The listing builds one solid part. Answer for the finished solid, in the listing's coordinates (mm). Face numbers are marked on the shaded views. A direction names the side the tool comes from. Round coordinates to 2 decimals unless told otherwise and drop trailing zeros. Write each loop counter-clockwise with the first axis right and the second up, starting at its lowest first coordinate (ties: lowest second). Pieces come first, ordered by that corner, then holes. Notation, with made-up numbers: (-6.75, 37.25) - (-1.75, 37.25) arc R31 cw to (-1.75, 64.25) - close; hole circle Ø2 at (20.25, 26.25). An arc over 180 degrees is marked (long way). Use a Markdown table: item, result. Add a question column.
1) A tool of negligible diameter and unlimited length cuts with its end or side. For the marked faces 1 and 2, from which of +Z, -Z, +X, -X, +Y, -Y can it reach the whole face along a straight path? Write none if from no direction.
2) Each of these flat-tipped pins is pushed along its axis until it touches: P1, Ø1, axis at x = 38.5, y = 7, coming from the +Z side; P2, Ø1.5, axis at y = 34, z = -273, coming from the +X side. Where does it stop, or does it pass through?
3) Find the intervals of material crossed by probe 1 along X at (y, z) = (30, -216); probe 2 along Z at (x, y) = (-120, 26.5) (3 decimals), in increasing order. Write a range as from..to.
4) A cutting plane is placed at A-A (x = -148). Give the vertices of the cut face in (y, z) (3 decimals), then the cut area to 3 significant figures.
5) A cutting plane is placed at B-B (z = -319.5). Give the vertices of the cut face in (x, y) (1 decimal), then the cut area to 3 significant figures.
```python
from build123d import *

# Parameters (mm, degrees)
SKETCH1_W           = 473.075
SKETCH1_H           = 95.25
BOSS_EXTRUDE1_DEPTH = 3.175
SKETCH3_W           = 78.74
SKETCH3_H           = 51.308
CUT_EXTRUDE2_DEPTH  = 242.305221983
SKETCH4_R           = 8.255
CUT_EXTRUDE3_DEPTH  = 242.305221983
SKETCH5_R           = 1.5875
CUT_EXTRUDE4_DEPTH  = 242.305221983
SKETCH6_W           = 3.175
SKETCH6_H           = 95.25
BOSS_EXTRUDE2_DEPTH = 377.825
SKETCH8_W           = 82.55
SKETCH8_H           = 33.324907577
CUT_EXTRUDE6_DEPTH  = 29.464
SKETCH9_R           = 3.175
CUT_EXTRUDE7_DEPTH  = 451.975752709


with BuildPart() as part:
    # Sketch1 → Boss-Extrude1 (new body)
    with BuildSketch(Plane.XY):
        Rectangle(SKETCH1_W, SKETCH1_H)
    extrude(amount=BOSS_EXTRUDE1_DEPTH)

    # Sketch3 → Cut-Extrude2 (cut, through all)
    with BuildSketch(Plane.XY.offset(3.175)):
        with Locations((0, 6.731)):
            Rectangle(SKETCH3_W, SKETCH3_H)
    extrude(amount=-CUT_EXTRUDE2_DEPTH, mode=Mode.SUBTRACT)

    # Sketch4 → Cut-Extrude3 (cut, through all)
    with BuildSketch(Plane.XY.offset(3.175)):
        with Locations((37.592, -35.814)):
            Circle(SKETCH4_R)
    extrude(amount=-CUT_EXTRUDE3_DEPTH, mode=Mode.SUBTRACT)

    # Sketch5 → Cut-Extrude4 (cut, through all)
    with BuildSketch(Plane.XY.offset(3.175)):
        with Locations((-44.196, 40.259)):
            Circle(SKETCH5_R)
        with Locations((44.196, 40.259)):
            Circle(SKETCH5_R)
        with Locations((-44.196, -24.765)):
            Circle(SKETCH5_R)
        with Locations((44.196, -24.765)):
            Circle(SKETCH5_R)
    extrude(amount=-CUT_EXTRUDE4_DEPTH, mode=Mode.SUBTRACT)

    # Sketch6 → Boss-Extrude2 (add)
    with BuildSketch(Plane(origin=(0, 0, 0), x_dir=(-1, 0, 0), z_dir=(0, 0, -1))):
        with Locations((234.95, 0)):
            Rectangle(SKETCH6_W, SKETCH6_H)
    extrude(amount=BOSS_EXTRUDE2_DEPTH)

    # Sketch8 → Cut-Extrude6 (cut)
    with BuildSketch(Plane.XY.offset(3.175)):
        with Locations((109.22, -30.962546212)):
            Rectangle(SKETCH8_W, SKETCH8_H)
        with BuildLine():
            Line((71.12, 14.274907577), (147.32, 14.274907577))
            ThreePointArc((147.32, 14.274907577), (150.495, 17.449907577), (147.32, 20.624907577))
            Line((147.32, 20.624907577), (71.12, 20.624907577))
            ThreePointArc((71.12, 20.624907577), (67.945, 17.449907577), (71.12, 14.274907577))
        make_face()
        with BuildLine():
            Line((-185.7375, 19.318625561), (-71.4375, 19.318625561))
            ThreePointArc((-71.4375, 19.318625561), (-68.2625, 22.493625561), (-71.4375, 25.668625561))
            Line((-71.4375, 25.668625561), (-185.7375, 25.668625561))
            ThreePointArc((-185.7375, 25.668625561), (-188.9125, 22.493625561), (-185.7375, 19.318625561))
        make_face()
        with BuildLine():
            Line((-185.7375, -6.081374439), (-71.4375, -6.081374439))
            ThreePointArc((-71.4375, -6.081374439), (-68.2625, -2.906374439), (-71.4375, 0.268625561))
            Line((-71.4375, 0.268625561), (-185.7375, 0.268625561))
            ThreePointArc((-185.7375, 0.268625561), (-188.9125, -2.906374439), (-185.7375, -6.081374439))
        make_face()
        with BuildLine():
            Line((-185.7375, -31.481374439), (-71.4375, -31.481374439))
            ThreePointArc((-71.4375, -31.481374439), (-68.2625, -28.306374439), (-71.4375, -25.131374439))
            Line((-71.4375, -25.131374439), (-185.7375, -25.131374439))
            ThreePointArc((-185.7375, -25.131374439), (-188.9125, -28.306374439), (-185.7375, -31.481374439))
        make_face()
    extrude(amount=-CUT_EXTRUDE6_DEPTH, mode=Mode.SUBTRACT)

    # Sketch9 → Cut-Extrude7 (cut, through all)
    with BuildSketch(Plane.XY.offset(3.175)):
        with Locations((181.715661459, 16.725735437)):
            Circle(SKETCH9_R)
        with Locations((193.599351225, 16.725735437)):
            Circle(SKETCH9_R)
        with Locations((204.910333051, 16.725735437)):
            Circle(SKETCH9_R)
    extrude(amount=-CUT_EXTRUDE7_DEPTH, mode=Mode.SUBTRACT)


solid = part.part
```
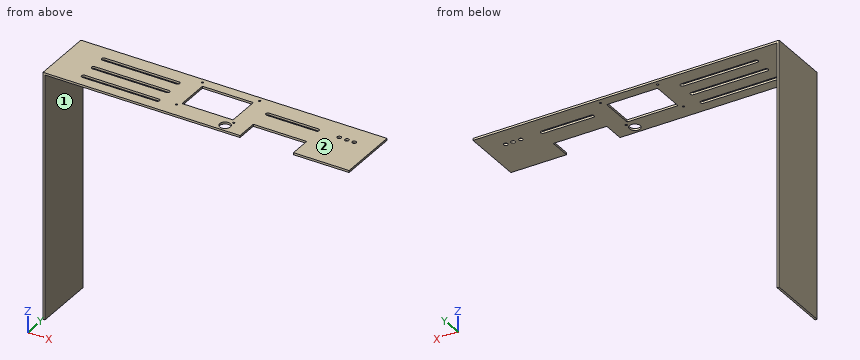
Entries:
| question | item | result |
|---|---|---|
| 1 | face 1 | -Z, +X, +Y, -Y |
| 1 | face 2 | +Z, +X, -X, +Y, -Y |
| 2 | P1 | passes through |
| 2 | P2 | stops at x = -233.36 |
| 3 | probe 1 | x = -236.54..-233.36 |
| 3 | probe 2 | z = 0..3.175 |
| 4 | outline | (-47.625, 0) - (-31.481, 0) - (-31.481, 3.175) - (-47.625, 3.175) - close; (-25.131, 0) - (-6.081, 0) - (-6.081, 3.175) - (-25.131, 3.175) - close; (0.269, 0) - (19.319, 0) - (19.319, 3.175) - (0.269, 3.175) - close; (25.669, 0) - (47.625, 0) - (47.625, 3.175) - (25.669, 3.175) - close |
| 4 | area | 242 mm² |
| 5 | outline | (-236.5, -47.6) - (-233.4, -47.6) - (-233.4, 47.6) - (-236.5, 47.6) - close |
| 5 | area | 302 mm² |
